Geometry: see drawing. Coordinates: mm, zero at the bounding-box minimum. A direction names the side the tool comes from. Round coordinates to 2 decimals unless told otherwise and drop trailing zeros. Order: outer loops, then holes, each group sorted by start corner. A loop starts at its lowest first (then second) coordinate and runs counter-clockwise, first axis right, second up. Notation, with made-up numbers: (24.5, 25.5) - (72.5, 25.5) arc R22 cw to (72.5, 55.5) - close; hole circle Ø7 at (47, 44). An arc over 180 degrees is marked (long way). Put each result on its own line as item: value. Start each with the question number.
1) Section D-D on z = 5. Output: boundary loops of the cut face in (x, y).
2) Mould query, pull axis X, two halves, no side actions, for the marked faces 3, 4 and 5. Classes: +X half, -X half, draft (parallel to the pull), parting line (faces both ways), or undercut.
3) Section B-B on x = 15. Output: boundary loops of the cut face in (y, z), then the cut area to 3 significant figures.
4) Section C-C on x = 5. Output: boundary loops of the cut face in (y, z), then the cut area to 3 significant figures.
5) Section A-A on z = 17. Output: boundary loops of the cut face in (x, y), then the cut area to 3 significant figures.
6) Contact query for a flat-ended pin moving along its axis: P1, Ø1.5, axis at x = 10, z = 25, coming from the +Y side. Output: stop coordinate, or through.
7) Access query for the marked faces 1 and 2. Directions: +Z, -Z, +X, -X, +Y, -Y. A direction counts if a zero-diameter tool reaches every point of the face in a straight line with its end or side. Return the directions, or none.
8) Line query: probe 1 along X at (y, z) = (4.75, 34) (1 decimal); probe 2 along Z at (x, y) = (26, 13.75); probe 3 along X at (y, z) = (6, 5). Output: solid intervals per line, ascending. Write a range as [from, to].
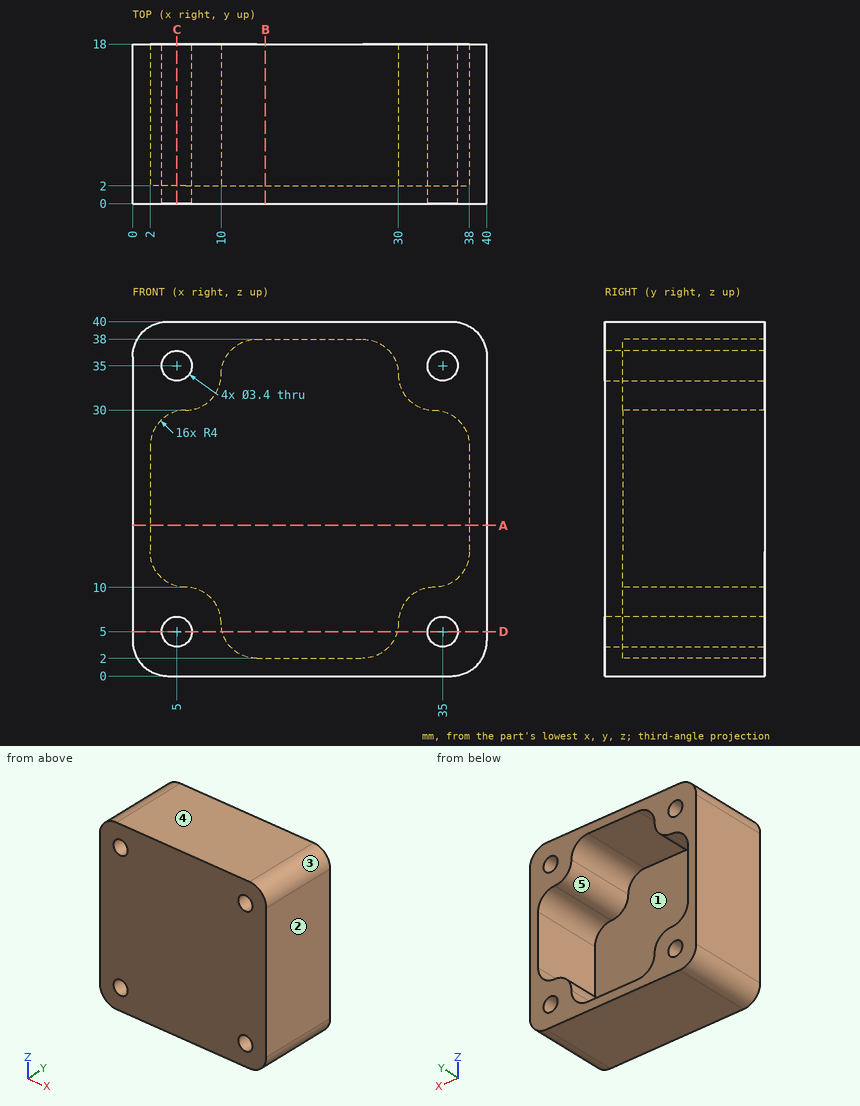
Answer sheet:
1. outline: (0, 0) - (3.3, 0) - (3.3, 18) - (0, 18) - close; (6.7, 0) - (33.3, 0) - (33.3, 18) - (29.87, 18) - (29.87, 2) - (10.13, 2) - (10.13, 18) - (6.7, 18) - close; (36.7, 0) - (40, 0) - (40, 18) - (36.7, 18) - close
2. face 3: +X half
2. face 4: draft
2. face 5: undercut
3. outline: (0, 0) - (18, 0) - (18, 2) - (2, 2) - (2, 38) - (18, 38) - (18, 40) - (0, 40) - close
3. area: 144 mm^2
4. outline: (0, 0) - (18, 0) - (18, 3.3) - (0, 3.3) - close; (0, 6.7) - (18, 6.7) - (18, 10.13) - (2, 10.13) - (2, 29.87) - (18, 29.87) - (18, 33.3) - (0, 33.3) - close; (0, 36.7) - (18, 36.7) - (18, 40) - (0, 40) - close
4. area: 282 mm^2
5. outline: (0, 0) - (40, 0) - (40, 18) - (38, 18) - (38, 2) - (2, 2) - (2, 18) - (0, 18) - close
5. area: 144 mm^2
6. P1: y = 2
7. face 1: +Y
7. face 2: +Z, -Z, +X, +Y, -Y
8. probe 1: [0, 3.6], [6.4, 10], [30, 33.6], [36.4, 40]
8. probe 2: [0, 2], [38, 40]
8. probe 3: [0, 3.3], [6.7, 10.13], [29.87, 33.3], [36.7, 40]
